Geometry check sheet. Reference: the model listing, model coordinates, mm. A direction names the side the tool comes from. Coordinates: 2 decimals unless noted, no trailing zeros. Order: outer loops, then holes, each group sorted by start corner. A loop starts at its lowest first (then second) coordinate and runs counter-clockwise, first axis right, second up. Notation, with made-up numbers: (44.5, -4) - (76.5, -4) arc R25 ccw to (76.5, 20) - close; hole circle Ø8 at (53, 88.25). An arc over 180 degrees is marked (long way). One line per item, written item: value. Start each with the question number.
```python
from build123d import *

# Parameters (mm, degrees)
F0_W     = 120
F0_H     = 70
F1_DEPTH = 10
F2_R     = 10
F3_DEPTH = 10.001
F4_DEPTH = 45
F6_DEPTH = 50


with BuildPart() as f1:
    # F0 (on Front) → F1 (new body)
    with BuildSketch(Plane.XZ):
        Rectangle(F0_W, F0_H)
    extrude(amount=F1_DEPTH)

    # F2 (on face) → F3 (cut, through all)
    with BuildSketch(Plane.XZ.offset(10)):
        with Locations((-45, 5)):
            Circle(F2_R)
        with Locations((44, 5)):
            Circle(F2_R)
    extrude(amount=-F3_DEPTH, mode=Mode.SUBTRACT)

    # F2 (on face) → F4 (join)
    with BuildSketch(Plane.XZ.offset(10)):
        Polygon((-15, 35), (-25, 35), (-25, -25), (-25, -35), (-15, -35), (15, -35), (25, -35), (25, -25), (25, 35), (15, 35), (15, -25), (-15, -25), align=None)
    extrude(amount=F4_DEPTH)

    # F5 (on face) → F6 (cut, through all)
    with BuildSketch(Plane.YZ.offset(25)):
        Polygon((-55, -25), (-20, 35), (-55, 35), align=None)
    extrude(amount=-F6_DEPTH, mode=Mode.SUBTRACT)


solid = f1.part
```
Q1. Set-up check for faces 1 (the flat face through (0, -10, 5)), 2 (the flat face through (-43, -10, -7)), 3 (the flat face through (-60, -5, 0)), 4 (the flat face through (42, -10, -7)): record each of +Z, -Z, +X, -X, +Y, -Y from which the full face is reachable in a straight line by a thin tool's end or side.
Q2. Release check for a two-part mould opening along Z. For faces 5 (the cylindrical face through (36.63, -5.07, 11.76)), 6 (the flat face through (25, -27, -8)), 7 (the flat face through (-1, -21, -35)) record: released by +Z, released by -Z, zero draft, split by the parting line, or undercut.
Q3. Cross-section at D-D, the plane y = -15.5. Enter the section's corners in (x, z).
Q4. Cross-section at A-A, the plane z = 5. Enter the section's corners in (x, y).
Q5. Material ranges on probe 1 along Z at (x, y) = (-45, -3); probe 2 along X at (y, z) = (-15, 27.5); probe 3 along Y at (x, z) = (-1.5, 23.5), recorded low to high.
Q6. Gauge pin test, flat ends, axial feed: P1, Ø8, axis at x = 19, z = 19.5, coming from the -Y side (3 decimals); P2, Ø13.5, axis at y = -24, z = -1, coming from the -X side; P3, Ø1.5, axis at x = -6, y = -14.5, coming from the +Z side; P4, Ø10.5, axis at x = 41, z = 3, coming from the -Y side. Record the tip position at first contact, or that the pin passes through.
Q7. Cross-section at B-B, the plane x = 44. Enter the section's corners in (y, z).
Q8. Cross-section at C-C, the plane z = 23. Enter the section's corners in (x, y).
Check result:
1. face 1: +Z, -Y
1. face 2: +Z, -Z, -X, -Y
1. face 3: +Z, -Z, -X, +Y, -Y
1. face 4: +Z, -Z, +X, -Y
2. face 5: undercut
2. face 6: zero draft
2. face 7: released by -Z
3. outline: (-25, -35) - (25, -35) - (25, 35) - (15, 35) - (15, -25) - (-15, -25) - (-15, 35) - (-25, 35) - close
4. outline: (-60, -10) - (-55, -10) - (-55, 0) - (-60, 0) - close; (-35, -10) - (-25, -10) - (-25, -37.5) - (-15, -37.5) - (-15, -10) - (15, -10) - (15, -37.5) - (25, -37.5) - (25, -10) - (34, -10) - (34, 0) - (-35, 0) - close; (54, -10) - (60, -10) - (60, 0) - (54, 0) - close
5. probe 1: z = -35 to -5, 15 to 35
5. probe 2: x = -25 to -15, 15 to 25
5. probe 3: y = -10 to 0
6. P1: stops at y = -31.375
6. P2: stops at x = -25
6. P3: stops at z = -25
6. P4: passes through
7. outline: (-10, -35) - (0, -35) - (0, -5) - (-10, -5) - close; (-10, 15) - (0, 15) - (0, 35) - (-10, 35) - close
8. outline: (-60, -10) - (-25, -10) - (-25, -27) - (-15, -27) - (-15, -10) - (15, -10) - (15, -27) - (25, -27) - (25, -10) - (60, -10) - (60, 0) - (-60, 0) - close
